from build123d import *

# Parameters (mm, degrees)
SKETCH1_W                                        = 111
SKETCH1_H                                        = 32
BOSS_EXTRUDE1_DEPTH                              = 14
BOSS_EXTRUDE2_DEPTH                              = 28
BOSS_EXTRUDE3_DEPTH                              = 14
BOSS_EXTRUDE3_DEPTH_BACK                         = 16
SKETCH1_4_R                                      = 16
F_18_0_18_DIAMETER_HOLE1_D                       = 18
CSK_FOR_M10_FLAT_HEAD_MACHINE_SCREW1_D           = 11
CSK_FOR_M10_FLAT_HEAD_MACHINE_SCREW1_CSINK_D     = 20
CSK_FOR_M10_FLAT_HEAD_MACHINE_SCREW1_CSINK_ANGLE = 90
BOSS_EXTRUDE5_DEPTH                              = 14
BOSS_EXTRUDE5_DEPTH_BACK                         = 46
SKETCH4_R                                        = 15
CUT_EXTRUDE2_DEPTH                               = 32
FILLET1_R                                        = 10


with BuildPart() as part:
    # Sketch1 → Boss-Extrude1 (new body)
    with BuildSketch(Plane(origin=(0, 0, 0), x_dir=(1, 0, 0), z_dir=(0, 1, 0))):
        with Locations((55.5, 16)):
            Rectangle(SKETCH1_W, SKETCH1_H)
    extrude(amount=BOSS_EXTRUDE1_DEPTH)

    # Sketch1<3> → Boss-Extrude2 (add)
    with BuildSketch(Plane(origin=(0, 0, 0), x_dir=(1, 0, 0), z_dir=(0, 1, 0))):
        with BuildLine():
            ThreePointArc((0, 32), (-16, 16), (0, 0))
            Line((0, 0), (0, 32))
        make_face()
        with BuildLine():
            Line((0, 32), (0, 0))
            ThreePointArc((0, 0), (11.313708499, 4.686291501), (16, 16))
            ThreePointArc((16, 16), (11.313708499, 27.313708499), (0, 32))
        make_face()
    extrude(amount=BOSS_EXTRUDE2_DEPTH)

    # Sketch1<4> → Boss-Extrude3 (add, two sides: drawn at the far end of the back side and taken through both)
    with BuildSketch(Plane(origin=(0, 0, 0), x_dir=(1, 0, 0), z_dir=(0, 1, 0)).offset(-BOSS_EXTRUDE3_DEPTH_BACK)):
        with Locations(Location((111, 16, 0), (0, 0, 270))):
            Circle(SKETCH1_4_R)
    extrude(amount=BOSS_EXTRUDE3_DEPTH + BOSS_EXTRUDE3_DEPTH_BACK)

    # Ø18.0 (18) Diameter Hole1 (through all)
    with Locations(Plane(origin=(0, 28, -16), x_dir=(0, 0, 1), z_dir=(0, 1, 0))):
        with Locations((0, 0)):
            Hole(F_18_0_18_DIAMETER_HOLE1_D / 2)

    # CSK for M10 Flat Head Machine Screw1 (through all)
    with Locations(Plane(origin=(111, 14, -16), x_dir=(0, 0, 1), z_dir=(0, 1, 0))):
        with Locations((0, 0)):
            CounterSinkHole(CSK_FOR_M10_FLAT_HEAD_MACHINE_SCREW1_D / 2, CSK_FOR_M10_FLAT_HEAD_MACHINE_SCREW1_CSINK_D / 2, counter_sink_angle=CSK_FOR_M10_FLAT_HEAD_MACHINE_SCREW1_CSINK_ANGLE)

    # Sketch4 → Boss-Extrude5 (add, two sides: drawn at the far end of the back side and taken through both)
    with BuildSketch(Plane.XY.offset(-BOSS_EXTRUDE5_DEPTH_BACK)):
        with Locations((55.5, 7)):
            Circle(SKETCH4_R)
        Polygon((64, 7), (59.75, 14.361215932), (51.25, 14.361215932), (47, 7), (51.25, -0.361215932), (59.75, -0.361215932), align=None, mode=Mode.SUBTRACT)
    extrude(amount=BOSS_EXTRUDE5_DEPTH + BOSS_EXTRUDE5_DEPTH_BACK)

    # Sketch4<3> → Cut-Extrude2 (cut)
    with BuildSketch(Plane.XY):
        Polygon((59.958548116, 0), (64, 7), (59.958548116, 14), (51.041451884, 14), (47, 7), (51.041451884, 0), align=None)
    extrude(amount=-CUT_EXTRUDE2_DEPTH, mode=Mode.SUBTRACT)

    # Fillet1
    fillet1_edges = [part.edges().sort_by_distance(p)[0] for p in [
        (42.233500839, 0, -16),
        (68.766499161, 0, -16),
        (68.766499161, 14, -16),
        (42.233500839, 14, -16),
    ]]
    fillet(fillet1_edges, radius=FILLET1_R)


solid = part.part
Geometry check sheet. Reference: the model listing, model coordinates, mm. A direction names the side the tool comes from. Give positions to 0.01 mm unless a question says otherwise; leave off trailing zeros. Loops run counter-clockwise (first coordinate to the right, second up) from the corner with the lowest first, then second, coordinate; pieces in that order, holes last. Notation, with made-up numbers: M 31.5,-25.75 L 64.5,-25.75 A20 cw 64.5,7.25 Z; hole C 51,-15.5 d11. An arc over 180 degrees is marked long. Answer as a JSON object with one key per item and string values. Group by question number.
Item 1: Sectioned sample at A-A on z = 8.5. Record the boundary of the cut face in (x, y).
Item 2: Material ranges on L1, parallel to X at y = -1, z = -16; L2, parallel to Z at x = 111, y = -1; L3, parallel to Y at x = 26.5, z = -22.5, recorded low to high.
Item 3: Gauge pin test, flat ends, axial feed: pin 1 (4 mm diameter, centred on y = 6.5, z = -24.5, fed in from -X); pin 2 (14.5 mm diameter, centred on x = 0, z = -16, fed in from -Y); pin 3 (4 mm diameter, centred on y = 6, z = -36, fed in from -X); pin 4 (1 mm diameter, centred on x = 28.5, y = 9.5, fed in from -Z). Record the tip position at first contact, or that the pin passes through.
Item 4: Access from +Z, -Z, +X, -X, +Y, -Y to the whole of each face (thin tool, end or side, straight path). Record for faces 4 (the flat face through (56, 14.361, -16)), 5 (the cylindrical face through (41.222, 14.858, -16.224)), 6 (the flat face through (95, 14, -16)).
Item 5: Sectioned sample at C-C on z = -13.5. Give the number of separate pieces and of enclosed holes in the cut face, plus the area to 3 significant figures.
Item 6: Mould release check, pull along Z, two halves, no side actions. Record for faces 1 (the cylindrical face through (116.453, -3.428, -15.284)), 2 (the cylindrical face through (62.42, -6.31, -16.42)), 3 (the flat face through (22, 7, 0)): pulls with the +Z half, pulls with the -Z half, needs draft (parallel to the pull), parting line crosses it, or undercut.
Item 7: Sectioned sample at B-B on x = 55.5. Record the boundary of the cut face in (y, z).
Item 8: Sectioned sample at D-D on x = 32.5. Record the boundary of the cut face in (y, z), plus the area to 3 significant figures.
Findings below:
{
 "1": {"outline": "C 55.5,7 d30; hole M 47,7 L 51.25,-0.36 L 59.75,-0.36 L 64,7 L 59.75,14.36 L 51.25,14.36 Z"},
 "2": {"L1": "41.53 to 69.47, 95 to 105.5, 116.5 to 127", "L2": "-32 to -21.5, -10.5 to 0", "L3": "0 to 14"},
 "3": {"pin 1": "x = -14.62", "pin 2": "through", "pin 3": "x = 40.5", "pin 4": "z = -32"},
 "4": {"face 4": "+Z, -Z", "face 5": "+Z, -Z, +Y", "face 6": "+Z, -Z, +X, +Y"},
 "5": {"separate pieces": "3", "enclosed holes": "1", "area": "2,270 mm2"},
 "6": {"face 1": "undercut", "face 2": "needs draft", "face 3": "pulls with the +Z half"},
 "7": {"outline": "M -8,-46 L -0.36,-46 L -0.36,14 L -8,14 Z; M 14.36,-46 L 22,-46 L 22,14 L 14.36,14 Z"},
 "8": {"outline": "M 0,-32 L 14,-32 L 14,0 L 0,0 Z", "area": "448 mm2"}
}
